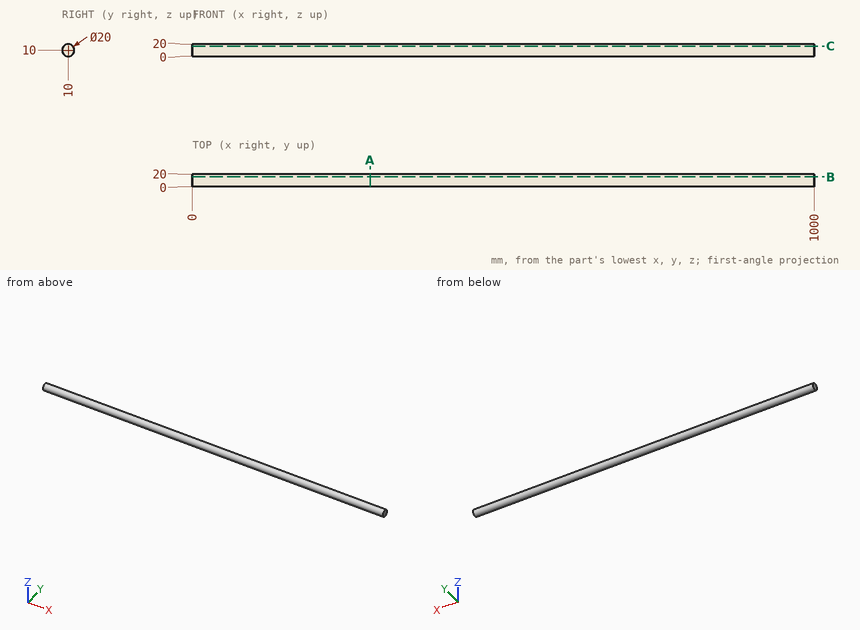
Geometry check sheet. Reference: drawing and pictorial views, mm from the part's lowest x, y, z. Give positions to 0.01 mm unless a question says otherwise; leave off trailing zeros. Loops run counter-clockwise (first coordinate to the right, second up) from the corner with the lowest first, then second, coordinate; pieces in that order, holes last. Notation, with made-up numbers: (-33, 55) - (5, 55) arc R24 ccw to (5, 65) - close; hole circle Ø1 at (-16.75, -6). An arc over 180 degrees is marked (long way). One line per question, with ' | ' between items. Start each with the question number.
1. Cross-section at A-A, the plane x = 286. Enter the section's corners in (y, z).
2. Gauge pin test, flat ends, axial feed: pin 1 Ø8 at (x, y) = (489, 16.5) entering from +Z; pin 2 Ø4 at (x, z) = (861.5, 10.5) entering from -Y; pin 3 Ø4 at (x, y) = (301, 16.5) entering from -Z; pin 4 Ø1 at (x, z) = (801, 9) entering from +Y. Record the tip position at first contact, or that the pin passes through.
3. Material ranges on line 1 along Y through (x, z) = (903.5, 8.25); line 2 along Y through (x, z) = (321, 10.75); line 3 along Z through (x, y) = (898.5, 13.75), recorded low to high. Write a range as [from, to].
4. Cross-section at B-B, the plane y = 16. Enter the section's corners in (x, z), plus the area to 3 significant figures.
5. Cross-section at C-C, the plane z = 16.5. Enter the section's corners in (x, y).
Check result:
1) outline: circle Ø20 at (10, 10)
2) pin 1: stops at z = 19.68 | pin 2: stops at y = 0 | pin 3: stops at z = 1.07 | pin 4: stops at y = 19.99
3) line 1: y = [0.15, 19.85] | line 2: y = [0.03, 19.97] | line 3: z = [0.73, 19.27]
4) outline: (0, 2) - (1000, 2) - (1000, 18) - (0, 18) - close | area: 16,000 mm2
5) outline: (0, 2.4) - (1000, 2.4) - (1000, 17.6) - (0, 17.6) - close
